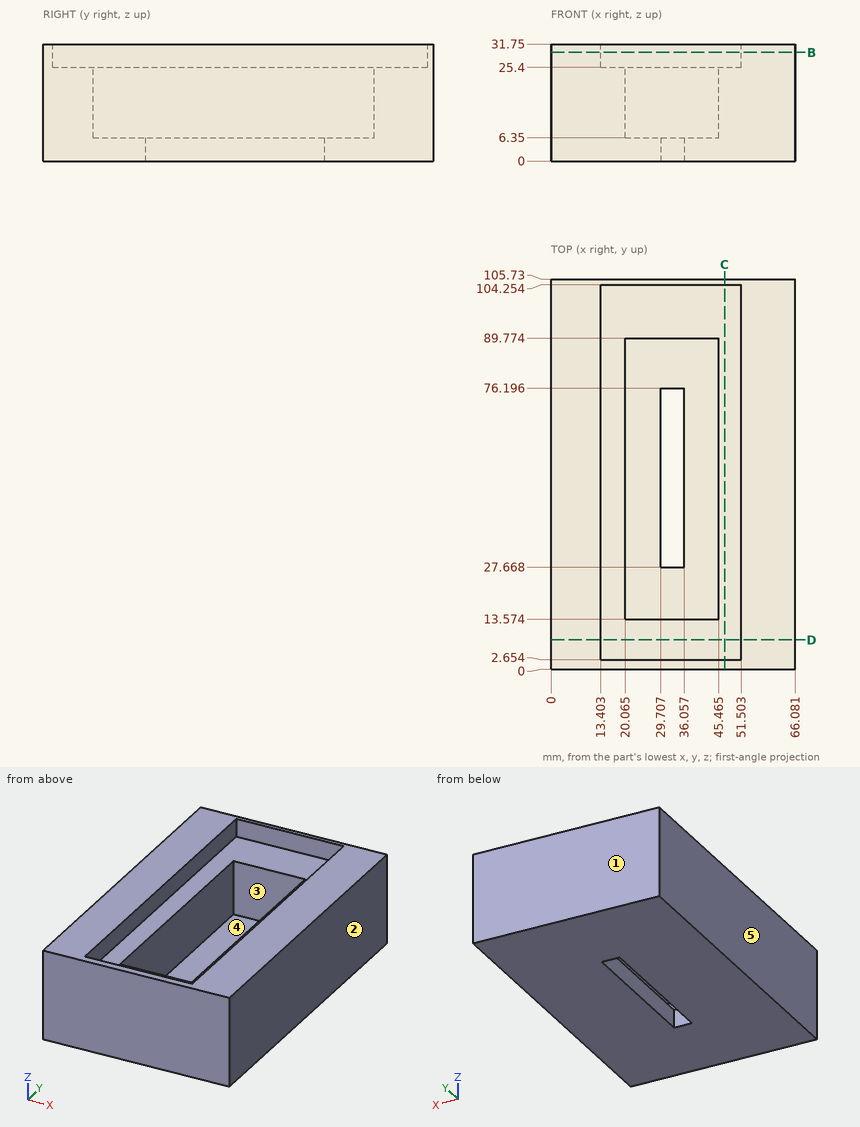
Design review of the part shown in the three views and the two pictorial views. Dimensions are in mm from the part's minimum x, y and z. A direction names the side the tool comes from. Give positions to 0.01 mm unless a question says otherwise; leave off trailing zeros. Write each loop counter-clockwise with the first axis right and the second up, starting at its lowest first coordinate (ties: lowest second). Pieces come first, ordered by that corner, then holes.
(1) Wall thickness on line 1 along X through (y, z) = (79, 27); line 2 along X through (y, z) = (65, 7) (1 decimal); line 3 along Y through (x, z) = (33.5, 24): over which ranges is each line inside the solid? List them lowest first.
Checked values:
line 1: x = 0 to 13.4, 51.5 to 66.08
line 2: x = 0 to 20.1, 45.5 to 66.1
line 3: y = 0 to 13.57, 89.77 to 105.73
(2) Add section B-B (z = 29.5). Give the boundary of the cut face in (x, y), and give its area (3 significant figures).
Checked values:
outline: (0, 0) - (66.08, 0) - (66.08, 105.73) - (0, 105.73) - close; hole (13.4, 2.65) - (51.5, 2.65) - (51.5, 104.25) - (13.4, 104.25) - close
area: 3,120 mm2
(3) Tool access review of the marked faces 4 and 5: name each direction out of +Z, -Z, +X, -X, +Y, -Y from which nothing blocks a thin tool from reaching the whole face with its end or side.
Checked values:
face 4: +Z
face 5: +Z, -Z, -X, +Y, -Y
(4) Add section D-D (y = 8). Give the boundary of the cut face in (x, z), and give its area (3 significant figures).
Checked values:
outline: (0, 0) - (66.08, 0) - (66.08, 31.75) - (51.5, 31.75) - (51.5, 25.4) - (13.4, 25.4) - (13.4, 31.75) - (0, 31.75) - close
area: 1,860 mm2
(5) Add section C-C (x = 47). Give the boundary of the cut face in (y, z), and give its area (3 significant figures).
Checked values:
outline: (0, 0) - (105.73, 0) - (105.73, 31.75) - (104.25, 31.75) - (104.25, 25.4) - (2.65, 25.4) - (2.65, 31.75) - (0, 31.75) - close
area: 2,710 mm2
(6) Mouldability with a two-part tool opening along Y and no side actions: class the marked faces 1, 2 and 3 as +Y half, -Y half, draft (parallel to the pull), parting line (faces both ways), or undercut.
Checked values:
face 1: +Y half
face 2: draft
face 3: undercut
(7) Clearance check with flat-ended pins moving along their axes: pin 1 Ø1 at (x, y) = (41, 82.5) entering from +Z; pin 2 Ø19 at (x, y) = (25, 47) entering from +Z. State where each tip first meets the part, or that it passes through.
Checked values:
pin 1: stops at z = 6.35
pin 2: stops at z = 25.4
